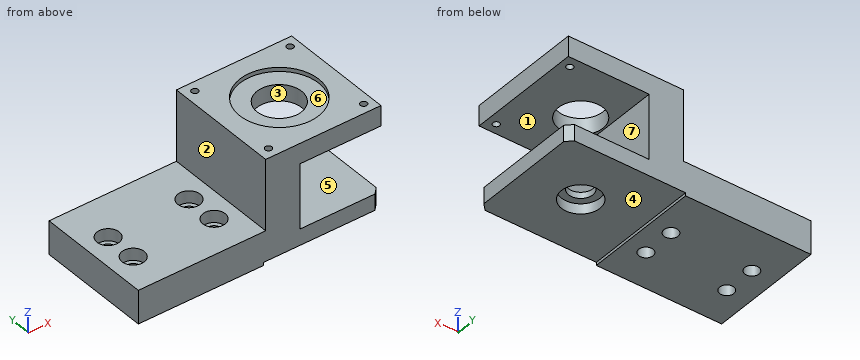
from build123d import *

# Parameters (mm, degrees)
SKETCH_1_W                   = 120
SKETCH_1_H                   = 57
EXTRUDE_1_DEPTH              = 50
SKETCH_2_W                   = 40
SKETCH_2_H                   = 32
CUT_EXTRUDE_1_DEPTH          = 142.947173272
SKETCH_3_W                   = 63
SKETCH_3_H                   = 35
CUT_EXTRUDE_2_DEPTH          = 142.947173272
SKETCH_4_W                   = 62
SKETCH_4_H                   = 57
EXTRUDE_2_DEPTH              = 1.5
SKETCH_5_R                   = 9.5
CUT_EXTRUDE_3_DEPTH          = 5
SKETCH_6_R                   = 6
CUT_EXTRUDE_4_DEPTH          = 20
SKETCH_7_R                   = 11
CUT_EXTRUDE_5_DEPTH          = 140.180638021
CHAMFER_1_SIZE               = 3
SKETCH_8_R                   = 19.5
CUT_EXTRUDE_6_DEPTH          = 2
HOLE_WIZARD_M6_1_D           = 7
HOLE_WIZARD_M6_1_CBORE_D     = 11
HOLE_WIZARD_M6_1_CBORE_DEPTH = 6
HOLE_WIZARD_M4_1_D           = 3.3
HOLE_WIZARD_M4_1_DEPTH       = 10.1
HOLE_WIZARD_M4_1_TIP         = 0.991420021


with BuildPart() as part:
    # 草图1 → 凸台-拉伸1 (new body)
    with BuildSketch(Plane.XY):
        with Locations((60, 28.5)):
            Rectangle(SKETCH_1_W, SKETCH_1_H)
    extrude(amount=EXTRUDE_1_DEPTH)

    # 草图2 → 切除-拉伸1 (cut, through all)
    with BuildSketch(Plane(origin=(0, 57, 0), x_dir=(1, 0, 0), z_dir=(0, 1, 0))):
        with Locations((100, -24)):
            Rectangle(SKETCH_2_W, SKETCH_2_H)
    extrude(amount=-CUT_EXTRUDE_1_DEPTH, mode=Mode.SUBTRACT)

    # 草图3 → 切除-拉伸2 (cut, through all)
    with BuildSketch(Plane(origin=(0, 57, 0), x_dir=(-1, 0, 0), z_dir=(0, 1, 0))):
        with Locations((-31.5, 32.5)):
            Rectangle(SKETCH_3_W, SKETCH_3_H)
    extrude(amount=-CUT_EXTRUDE_2_DEPTH, mode=Mode.SUBTRACT)

    # 草图4 → 凸台-拉伸2 (add)
    with BuildSketch(Plane(origin=(0, 0, 0), x_dir=(-1, 0, 0), z_dir=(0, 0, -1))):
        with Locations((-31, 28.5)):
            Rectangle(SKETCH_4_W, SKETCH_4_H)
    extrude(amount=EXTRUDE_2_DEPTH)

    # 草图5 → 切除-拉伸3 (cut)
    with BuildSketch(Plane(origin=(0, 0, 0), x_dir=(-1, 0, 0), z_dir=(0, 0, -1))):
        with Locations((-91.8, 28.5)):
            Circle(SKETCH_5_R)
    extrude(amount=-CUT_EXTRUDE_3_DEPTH, mode=Mode.SUBTRACT)

    # 草图6 → 切除-拉伸4 (cut)
    with BuildSketch(Plane(origin=(0, 0, 5), x_dir=(-1, 0, 0), z_dir=(0, 0, -1))):
        with Locations((-91.8, 28.5)):
            Circle(SKETCH_6_R)
    extrude(amount=-CUT_EXTRUDE_4_DEPTH, mode=Mode.SUBTRACT)

    # 草图7 → 切除-拉伸5 (cut, through all)
    with BuildSketch(Plane(origin=(0, 0, 40), x_dir=(-1, 0, 0), z_dir=(0, 0, -1))):
        with Locations((-91.8, 28.5)):
            Circle(SKETCH_7_R)
    extrude(amount=-CUT_EXTRUDE_5_DEPTH, mode=Mode.SUBTRACT)

    # 倒角1
    chamfer_1_edges = [part.edges().sort_by_distance(p)[0] for p in [
        (120, 0, 4),
        (120, 57, 4),
    ]]
    chamfer(chamfer_1_edges, length=CHAMFER_1_SIZE)

    # 草图8 → 切除-拉伸6 (cut)
    with BuildSketch(Plane.XY.offset(50)):
        with Locations((91.8, 28.5)):
            Circle(SKETCH_8_R)
    extrude(amount=-CUT_EXTRUDE_6_DEPTH, mode=Mode.SUBTRACT)

    # M6 六角凹头螺钉的柱形沉头孔1 (through all)
    with Locations(Plane.XY.offset(15)):
        with Locations((11.8, 34.5), (11.8, 18.5), (51.8, 18.5), (51.8, 34.5)):
            CounterBoreHole(HOLE_WIZARD_M6_1_D / 2, HOLE_WIZARD_M6_1_CBORE_D / 2, HOLE_WIZARD_M6_1_CBORE_DEPTH)

    # M4 螺纹孔1
    with Locations(Plane.XY.offset(50)):
        with Locations((68.25, 52), (115.35, 5), (115.35, 52), (68.25, 5)):
            Hole(HOLE_WIZARD_M4_1_D / 2, depth=HOLE_WIZARD_M4_1_DEPTH)
            with Locations((0, 0, -(HOLE_WIZARD_M4_1_DEPTH + HOLE_WIZARD_M4_1_TIP / 2))):  # 118° drill point
                Cone(0, HOLE_WIZARD_M4_1_D / 2, HOLE_WIZARD_M4_1_TIP, mode=Mode.SUBTRACT)


solid = part.part
The model under review builds one solid part; all positions refer to its coordinate system, in mm. Face numbers are marked on the shaded views. A direction names the side the tool comes from. Round coordinates to 2 decimals unless told otherwise and drop trailing zeros. Loops run counter-clockwise (first coordinate to the right, second up) from the corner with the lowest first, then second, coordinate; pieces in that order, holes last. Notation, with made-up numbers: (85, 48) -> (114, 48) arc R24 ccw to (114, 78) -> close; hole circle Ø8 at (15.25, -26.5). An arc over 180 degrees is marked (long way). Return JSON: item names as keys, results as strings.
(1) For the marked faces 1, 2, 3 and 4, list the 3-axis set-ups (+Z, -Z, +X, -X, +Y, -Y) from which the entire face can be reached by the end or side of a thin tool; tool diameter is ignored.
Solved:
{"face 1": "+X, +Y, -Y", "face 2": "+Z, -X, +Y, -Y", "face 3": "+Z", "face 4": "-Z, +X, +Y, -Y"}
(2) For pin 1 (21 mm diameter, centred on x = 92.5, y = 28.5, fed in from -Z); pin 2 (5 mm diameter, centred on y = 10.5, z = 26.5, fed in from +X); pin 3 (12 mm diameter, centred on x = 13, y = 35, fed in from +Z); pin 4 (6.5 mm diameter, centred on x = 51.8, y = 18.5, fed in from -Z), all flat-tipped, find the tip position at first contact; note any pin that passes through.
Solved:
{"pin 1": "z = 0", "pin 2": "x = 80", "pin 3": "z = 15", "pin 4": "through"}
(3) Add section A-A on x = 11.8. Write out the cut boundary in (y, z), plus the area to 4 significant figures.
Solved:
{"outline": "(0, -1.5) -> (15, -1.5) -> (15, 9) -> (13, 9) -> (13, 15) -> (0, 15) -> close; (22, -1.5) -> (31, -1.5) -> (31, 9) -> (29, 9) -> (29, 15) -> (24, 15) -> (24, 9) -> (22, 9) -> close; (38, -1.5) -> (57, -1.5) -> (57, 15) -> (40, 15) -> (40, 9) -> (38, 9) -> close", "area": "661.5 mm2"}
(4) For line 1 (Y direction, x = 115.35, z = 47.25); line 2 (Y direction, x = 11.8, z = 12.3); line 3 (X direction, y = 28, z = 49), list the stretches that pass through material, from the lowest coordinate up.
Solved:
{"line 1": "0 to 3.35, 6.65 to 50.35, 53.65 to 57", "line 2": "0 to 13, 24 to 29, 40 to 57", "line 3": "63 to 72.31, 111.29 to 120"}
(5) Add section C-C on z = 6.5. Write out the cut boundary in (x, y).
Solved:
{"outline": "(0, 0) -> (117, 0) -> (120, 3) -> (120, 54) -> (117, 57) -> (0, 57) -> close; hole circle Ø7 at (11.8, 18.5); hole circle Ø7 at (11.8, 34.5); hole circle Ø7 at (51.8, 18.5); hole circle Ø7 at (51.8, 34.5); hole circle Ø12 at (91.8, 28.5)"}
(6) Add section B-B on z = 45. Write out the cut boundary in (x, y).
Solved:
{"outline": "(63, 0) -> (120, 0) -> (120, 57) -> (63, 57) -> close; hole circle Ø3.3 at (68.25, 5); hole circle Ø3.3 at (68.25, 52); hole circle Ø22 at (91.8, 28.5); hole circle Ø3.3 at (115.35, 5); hole circle Ø3.3 at (115.35, 52)"}
(7) The part is to be moulded in two halves that separate along X. For the marked faces 5, 6 and 7, say which applies: released by +X, released by -X, zero draft, split by the parting line, or undercut.
Solved:
{"face 5": "zero draft", "face 6": "undercut", "face 7": "released by +X"}
(8) Add section D-D on x = 40.5. Write out the cut boundary in (y, z), plus the area to 4 significant figures.
Solved:
{"outline": "(0, -1.5) -> (57, -1.5) -> (57, 15) -> (0, 15) -> close", "area": "940.5 mm2"}
